Model file for the job. Use its own axes, mm. A direction names the side the tool comes from. Give positions to 0.01 mm unless a question says otherwise; leave off trailing zeros. Order: outer loops, then holes, each group sorted by start corner. A loop starts at its lowest first (then second) coordinate and runs counter-clockwise, first axis right, second up. Notation, with made-up numbers: M 2,10 L 48,10 A29 cw 48,35 Z; hole C 33,51.5 d11. An arc over 180 degrees is marked long. Return JSON: item names as keys, results as strings. Group by question number.
1. Slice it at C-C on x = 9.25. List the corners of the cut face in (y, z), then the cut area to 3 significant figures.
2. Pin check, flat tips, straight feed: pin 1 (4 mm diameter, centred on x = 9, z = 2, fed in from +Y); pin 2 (2.5 mm diameter, centred on x = 12, z = 0, fed in from -Y). Stop position of each tip, or through.
3. Wall check: probe 1 along X at (y, z) = (3.5, -3.5); probe 2 along Y at (x, z) = (-3.5, -3); probe 3 along X at (y, z) = (4.75, -5.5). Give the ranges that are in metal, low to high. Write a range as [from, to].
4. Slice it at B-B on x = -3. List the corners of the cut face in (y, z), then the cut area to 3 significant figures.
5. Slice it at D-D on z = 1. Give the number of separate pieces and of enclosed holes in the cut face, then the cut area to 3 significant figures.
6. Two-plate mould, pull along Z, no slides. Class faces 1 (the face through (0.02, -2.55, 0.02)), 2 (the face through (3.595, -2.461, 1.417)): released by +Z, released by -Z, zero draft, split by the parting line, or undercut.
7. Slice it at A-A on y = 0. List the corners of the cut face in (x, z), then the cut area to 3 significant figures.
8. 3-axis set-ups, long thin cutter, end or side, ignore diameter. For faces 3 (the face through (-3.863, 2, 0)), 4 (the face through (0, 6.5, 0)): which of +Z, -Z, +X, -X, +Y, -Y reach the whole face in a straight line?
from build123d import *

# Parameters (mm, degrees)
F1_DEPTH  = 6
F3_DEPTH  = 10
F4_W      = 10.5
F4_H      = 12
F4_R      = 2.55
F5_DEPTH  = 8
F1_FACE_R = 2.55
F6_DEPTH  = 8.6566


with BuildPart() as f1:
    # F0 (on Top) → F1 (new body, symmetric)
    with BuildSketch(Plane.XY):
        with BuildLine():
            Line((6.5, -5.25), (6.5, 5.25))
            ThreePointArc((6.5, 5.25), (6.133883, 6.133883), (5.25, 6.5))
            Line((5.25, 6.5), (-5.25, 6.5))
            ThreePointArc((-5.25, 6.5), (-6.133883, 6.133883), (-6.5, 5.25))
            Line((-6.5, 5.25), (-6.5, -5.25))
            ThreePointArc((-6.5, -5.25), (-6.133883, -6.133883), (-5.25, -6.5))
            Line((-5.25, -6.5), (5.25, -6.5))
            ThreePointArc((5.25, -6.5), (6.133883, -6.133883), (6.5, -5.25))
        make_face()
    extrude(amount=F1_DEPTH, both=True)

    # F2 (on Top) → F3 (cut, symmetric)
    with BuildSketch(Plane.XY):
        with BuildLine():
            ThreePointArc((0.889914, -2.1566), (0.928239, -2.163918), (0.961171, -2.184843))
            Line((0.961171, -2.184843), (2.745753, -3.863205))
            Line((2.745753, -3.863205), (1.752595, -3.863205))
            ThreePointArc((1.752595, -3.863205), (1.466924, -3.981534), (1.348595, -4.267205))
            Line((1.348595, -4.267205), (1.348595, -4.749805))
            ThreePointArc((1.348595, -4.749805), (1.466924, -5.035476), (1.752595, -5.153805))
            Line((1.752595, -5.153805), (4.749795, -5.153805))
            ThreePointArc((4.749795, -5.153805), (5.035466, -5.035476), (5.153795, -4.749805))
            Line((5.153795, -4.749805), (5.153795, -1.752605))
            ThreePointArc((5.153795, -1.752605), (5.035471, -1.466932), (4.749802, -1.348599))
            Line((4.749802, -1.348599), (4.267202, -1.348599))
            ThreePointArc((4.267202, -1.348599), (3.981531, -1.466927), (3.863202, -1.752599))
            Line((3.863202, -1.752599), (3.863202, -2.745756))
            Line((3.863202, -2.745756), (2.184831, -0.961164))
            ThreePointArc((2.184831, -0.961164), (2.163912, -0.928237), (2.156595, -0.889919))
            Line((2.156595, -0.889919), (2.156595, 0.889909))
            ThreePointArc((2.156595, 0.889909), (2.163912, 0.928229), (2.184834, 0.961157))
            Line((2.184834, 0.961157), (3.863202, 2.745746))
            Line((3.863202, 2.745746), (3.863202, 1.752589))
            ThreePointArc((3.863202, 1.752589), (3.981531, 1.466917), (4.267202, 1.348589))
            Line((4.267202, 1.348589), (4.749802, 1.348589))
            ThreePointArc((4.749802, 1.348589), (5.035473, 1.466917), (5.153802, 1.752589))
            Line((5.153802, 1.752589), (5.153802, 4.749789))
            ThreePointArc((5.153802, 4.749789), (5.035477, 5.035475), (4.749794, 5.153807))
            Line((4.749794, 5.153807), (1.752594, 5.153807))
            ThreePointArc((1.752594, 5.153807), (1.466922, 5.035478), (1.348594, 4.749807))
            Line((1.348594, 4.749807), (1.348594, 4.267207))
            ThreePointArc((1.348594, 4.267207), (1.466922, 3.981536), (1.752594, 3.863207))
            Line((1.752594, 3.863207), (2.745751, 3.863207))
            Line((2.745751, 3.863207), (0.961159, 2.184836))
            ThreePointArc((0.961159, 2.184836), (0.928232, 2.163916), (0.889914, 2.1566))
            Line((0.889914, 2.1566), (-0.889914, 2.1566))
            ThreePointArc((-0.889914, 2.1566), (-0.928238, 2.163918), (-0.961169, 2.184841))
            Line((-0.961169, 2.184841), (-2.745757, 3.863209))
            Line((-2.745757, 3.863209), (-1.7526, 3.863209))
            ThreePointArc((-1.7526, 3.863209), (-1.466929, 3.981538), (-1.3486, 4.267209))
            Line((-1.3486, 4.267209), (-1.3486, 4.749809))
            ThreePointArc((-1.3486, 4.749809), (-1.466937, 5.035473), (-1.752607, 5.153794))
            Line((-1.752607, 5.153794), (-4.749807, 5.153794))
            ThreePointArc((-4.749807, 5.153794), (-5.035478, 5.035465), (-5.153807, 4.749794))
            Line((-5.153807, 4.749794), (-5.153807, 1.752594))
            ThreePointArc((-5.153807, 1.752594), (-5.035478, 1.466922), (-4.749807, 1.348594))
            Line((-4.749807, 1.348594), (-4.267207, 1.348594))
            ThreePointArc((-4.267207, 1.348594), (-3.981536, 1.466922), (-3.863207, 1.752594))
            Line((-3.863207, 1.752594), (-3.863207, 2.745751))
            Line((-3.863207, 2.745751), (-2.184836, 0.961159))
            ThreePointArc((-2.184836, 0.961159), (-2.163916, 0.928232), (-2.1566, 0.889914))
            Line((-2.1566, 0.889914), (-2.1566, -0.889914))
            ThreePointArc((-2.1566, -0.889914), (-2.163918, -0.928238), (-2.184841, -0.961169))
            Line((-2.184841, -0.961169), (-3.863209, -2.745757))
            Line((-3.863209, -2.745757), (-3.863209, -1.7526))
            ThreePointArc((-3.863209, -1.7526), (-3.981538, -1.466929), (-4.267209, -1.3486))
            Line((-4.267209, -1.3486), (-4.749809, -1.3486))
            ThreePointArc((-4.749809, -1.3486), (-5.035481, -1.466929), (-5.153809, -1.7526))
            Line((-5.153809, -1.7526), (-5.153809, -4.7498))
            ThreePointArc((-5.153809, -4.7498), (-5.035481, -5.035471), (-4.749809, -5.1538))
            Line((-4.749809, -5.1538), (-1.752609, -5.1538))
            ThreePointArc((-1.752609, -5.1538), (-1.466938, -5.035471), (-1.348609, -4.7498))
            Line((-1.348609, -4.7498), (-1.348609, -4.2672))
            ThreePointArc((-1.348609, -4.2672), (-1.466935, -3.981539), (-1.752594, -3.863207))
            Line((-1.752594, -3.863207), (-2.745751, -3.863207))
            Line((-2.745751, -3.863207), (-0.961159, -2.184836))
            ThreePointArc((-0.961159, -2.184836), (-0.928232, -2.163916), (-0.889914, -2.1566))
            Line((-0.889914, -2.1566), (0.889914, -2.1566))
        make_face()
    extrude(amount=F3_DEPTH, both=True, mode=Mode.SUBTRACT)

    # F4 (on face) → F5 (join)
    with BuildSketch(Plane.YZ.offset(6.5)):
        Rectangle(F4_W, F4_H)
        Circle(F4_R, mode=Mode.SUBTRACT)
    extrude(amount=F5_DEPTH)

    # F1_face (on face) → F6 (cut, through all)
    with BuildSketch(Plane.YZ.offset(6.5)):
        Circle(F1_FACE_R)
    extrude(amount=-F6_DEPTH, mode=Mode.SUBTRACT)


solid = f1.part
Result:
{
 "1": {"outline": "M -5.25,-6 L 5.25,-6 L 5.25,6 L -5.25,6 Z; hole C 0,0 d5.1", "area": "106 mm2"},
 "2": {"pin 1": "stops at y = 5.25", "pin 2": "stops at y = -5.25"},
 "3": {"probe 1": "x = [-6.5, -5.15], [-2.36, 2.36], [5.15, 14.5]", "probe 2": "y = [-6.5, -5.15], [-2.36, 2.36], [5.15, 6.5]", "probe 3": "x = [-6.5, -5.15], [-1.35, 1.35], [5.15, 14.5]"},
 "4": {"outline": "M -6.5,-6 L -5.15,-6 L -5.15,6 L -6.5,6 Z; M -1.83,-6 L 1.83,-6 L 1.83,6 L -1.83,6 Z; M 5.15,-6 L 6.5,-6 L 6.5,6 L 5.15,6 Z", "area": "76.2 mm2"},
 "5": {"separate pieces": "3", "enclosed holes": "0", "area": "131 mm2"},
 "6": {"face 1": "undercut", "face 2": "zero draft"},
 "7": {"outline": "M -6.5,-6 L -2.16,-6 L -2.16,6 L -6.5,6 Z; M 2.16,-6 L 14.5,-6 L 14.5,-2.55 L 2.16,-2.55 Z; M 2.16,2.55 L 14.5,2.55 L 14.5,6 L 2.16,6 Z", "area": "137 mm2"},
 "8": {"face 3": "+Z, -Z", "face 4": "+Z, -Z, +X, -X, +Y"}
}
